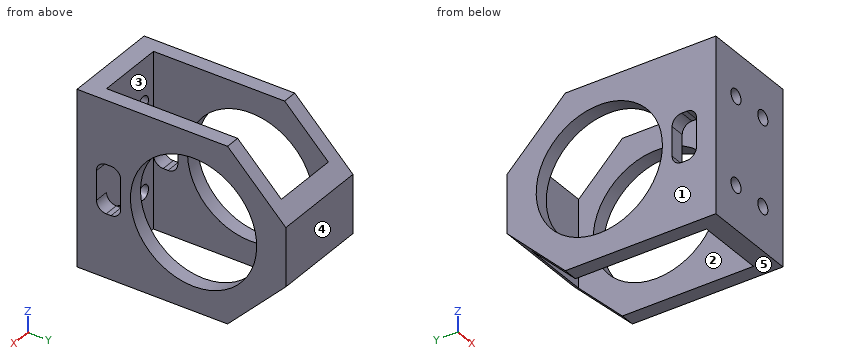
from build123d import *

# Parameters (mm, degrees)
SKETCH_1_W          = 20
SKETCH_1_H          = 36
EXTRUDE_1_DEPTH     = 4
SKETCH_2_W          = 3
SKETCH_2_H          = 36
EXTRUDE_2_DEPTH     = 36
SKETCH_3_W          = 20
SKETCH_3_H          = 36
EXTRUDE_3_DEPTH     = 3
SKETCH_4_R          = 13
CUT_EXTRUDE_1_DEPTH = 51.724747412
CUT_EXTRUDE_2_DEPTH = 51.724747412
SKETCH_6_R          = 1.5
CUT_EXTRUDE_3_DEPTH = 4
SKETCH_7_W          = 10
SKETCH_7_H          = 5
CUT_EXTRUDE_4_DEPTH = 51.724747412
FILLET_1_R          = 2


with BuildPart() as part:
    # 草图1 → 凸台-拉伸1 (new body)
    with BuildSketch(Plane(origin=(0, 0, 0), x_dir=(1, 0, 0), z_dir=(0, 1, 0))):
        Rectangle(SKETCH_1_W, SKETCH_1_H)
    extrude(amount=EXTRUDE_1_DEPTH)

    # 草图2 → 凸台-拉伸2 (add)
    with BuildSketch(Plane(origin=(0, 4, 0), x_dir=(1, 0, 0), z_dir=(0, 1, 0))):
        with Locations((-8.5, 0)):
            Rectangle(SKETCH_2_W, SKETCH_2_H)
        with Locations((8.5, 0)):
            Rectangle(SKETCH_2_W, SKETCH_2_H)
    extrude(amount=EXTRUDE_2_DEPTH)

    # 草图3 → 凸台-拉伸3 (add)
    with BuildSketch(Plane(origin=(0, 40, 0), x_dir=(1, 0, 0), z_dir=(0, 1, 0))):
        Rectangle(SKETCH_3_W, SKETCH_3_H)
    extrude(amount=EXTRUDE_3_DEPTH)

    # 草图4 → 切除-拉伸1 (cut, through all)
    with BuildSketch(Plane(origin=(10, 0, 0), x_dir=(0, 0, -1), z_dir=(1, 0, 0))):
        with Locations((0, 24)):
            Circle(SKETCH_4_R)
    extrude(amount=-CUT_EXTRUDE_1_DEPTH, mode=Mode.SUBTRACT)

    # 草图5 → 切除-拉伸2 (cut, through all)
    with BuildSketch(Plane(origin=(10, 0, 0), x_dir=(0, 0, -1), z_dir=(1, 0, 0))):
        Polygon((-6, 43), (-18, 31), (-18, 43), align=None)
        Polygon((18, 31), (18, 43), (6, 43), align=None)
    extrude(amount=-CUT_EXTRUDE_2_DEPTH, mode=Mode.SUBTRACT)

    # 草图6 → 切除-拉伸3 (cut)
    with BuildSketch(Plane(origin=(0, 4, 0), x_dir=(1, 0, 0), z_dir=(0, 1, 0))):
        with Locations(Location((4, 9, 0), (0, 0, 270))):
            Circle(SKETCH_6_R)
        with Locations(Location((-4, 9, 0), (0, 0, 90))):
            Circle(SKETCH_6_R)
        with Locations(Location((4, -9, 0), (0, 0, 90))):
            Circle(SKETCH_6_R)
        with Locations(Location((-4, -9, 0), (0, 0, 270))):
            Circle(SKETCH_6_R)
    extrude(amount=-CUT_EXTRUDE_3_DEPTH, mode=Mode.SUBTRACT)

    # 草图7 → 切除-拉伸4 (cut, through all)
    with BuildSketch(Plane(origin=(10, 0, 0), x_dir=(0, 0, -1), z_dir=(1, 0, 0))):
        with Locations((0, 6.5)):
            Rectangle(SKETCH_7_W, SKETCH_7_H)
    extrude(amount=-CUT_EXTRUDE_4_DEPTH, mode=Mode.SUBTRACT)

    # 圆角1
    fillet_1_edges = [part.edges().sort_by_distance(p)[0] for p in [
        (-8.5, 4, 5),
        (8.5, 4, 5),
        (-8.5, 9, 5),
        (8.5, 9, 5),
        (-8.5, 9, -5),
        (8.5, 9, -5),
        (-8.5, 4, -5),
        (8.5, 4, -5),
    ]]
    fillet(fillet_1_edges, radius=FILLET_1_R)


solid = part.part
Build history of the part. All positions in model axes, mm. Face numbers are marked on the shaded views. A direction names the side the tool comes from. Coordinates: 2 decimals unless noted, no trailing zeros. Order: outer loops, then holes, each group sorted by start corner. A loop starts at its lowest first (then second) coordinate and runs counter-clockwise, first axis right, second up. Notation, with made-up numbers: (-23, 11.5) - (-15, 11.5) arc R15 cw to (-15, 15.5) - close; hole circle Ø8 at (82.5, 85). An arc over 180 degrees is marked (long way). Put each result on its own line as item: value.
1. Saw through at A-A (x = -0.5). Write the cut outline in (y, z).
Answer sheet:
outline: (0, -18) - (4, -18) - (4, 18) - (0, 18) - close; (40, -9) - (43, -6) - (43, 6) - (40, 9) - close
2. Saw through at D-D (x = -4). Write the cut outline in (y, z).
Answer sheet:
outline: (0, -18) - (4, -18) - (4, -10.5) - (0, -10.5) - close; (0, -7.5) - (4, -7.5) - (4, 7.5) - (0, 7.5) - close; (0, 10.5) - (4, 10.5) - (4, 18) - (0, 18) - close; (40, -9) - (43, -6) - (43, 6) - (40, 9) - close
3. Saw through at B-B (y = 12). Write the cut outline in (x, z).
Answer sheet:
outline: (-10, -18) - (-7, -18) - (-7, -5) - (-10, -5) - close; (-10, 5) - (-7, 5) - (-7, 18) - (-10, 18) - close; (7, -18) - (10, -18) - (10, -5) - (7, -5) - close; (7, 5) - (10, 5) - (10, 18) - (7, 18) - close
4. Saw through at C-C (z = 0). Write the cut outline in (x, y), and give its area (3 significant figures).
Answer sheet:
outline: (-10, 0) - (10, 0) - (10, 4) - (-10, 4) - close; (-10, 9) - (-7, 9) - (-7, 11) - (-10, 11) - close; (-10, 37) - (-7, 37) - (-7, 40) - (7, 40) - (7, 37) - (10, 37) - (10, 43) - (-10, 43) - close; (7, 9) - (10, 9) - (10, 11) - (7, 11) - close
area: 170 mm^2
5. Probe line 1 along X through (y, z) = (2.25, -9); line 2 along Y through (x, z) = (-8.2, 0); line 3 along X through (y, z) = (33, -14). List the from-to ranges inside material, lowest first. Write a range as [from, to].
Answer sheet:
line 1: x = [-10, -5.5], [-2.5, 2.5], [5.5, 10]
line 2: y = [0, 4], [9, 11], [37, 43]
line 3: x = [-10, -7], [7, 10]
6. Tool access for the marked faces 1 and 2: list every direction of +Z, -Z, +X, -X, +Y, -Y with a clear straight run to the whole face (end or side of a thin tool).
Answer sheet:
face 1: +Z, -Z, -X, +Y, -Y
face 2: +Z, -Z
7. Pull direction Y, two halves, no side cores. Call the marked faces 3, 4 and 5: pulls with the +Y half, pulls with the -Y half, needs draft (parallel to the pull), parting line crosses it, or undercut.
Answer sheet:
face 3: undercut
face 4: pulls with the +Y half
face 5: needs draft
8. Drop flat-ended pins along their axis: P1, Ø3, axis at x = 3, z = 13, coming from the +Y side; P2, Ø1.8, axis at x = 4, z = 9, coming from the -Y side; P3, Ø4, axis at x = 1, z = 2, coming from the -Y side. Give the stop position or say it passes through.
Answer sheet:
P1: stops at y = 4
P2: stops at y = 40
P3: stops at y = 0
